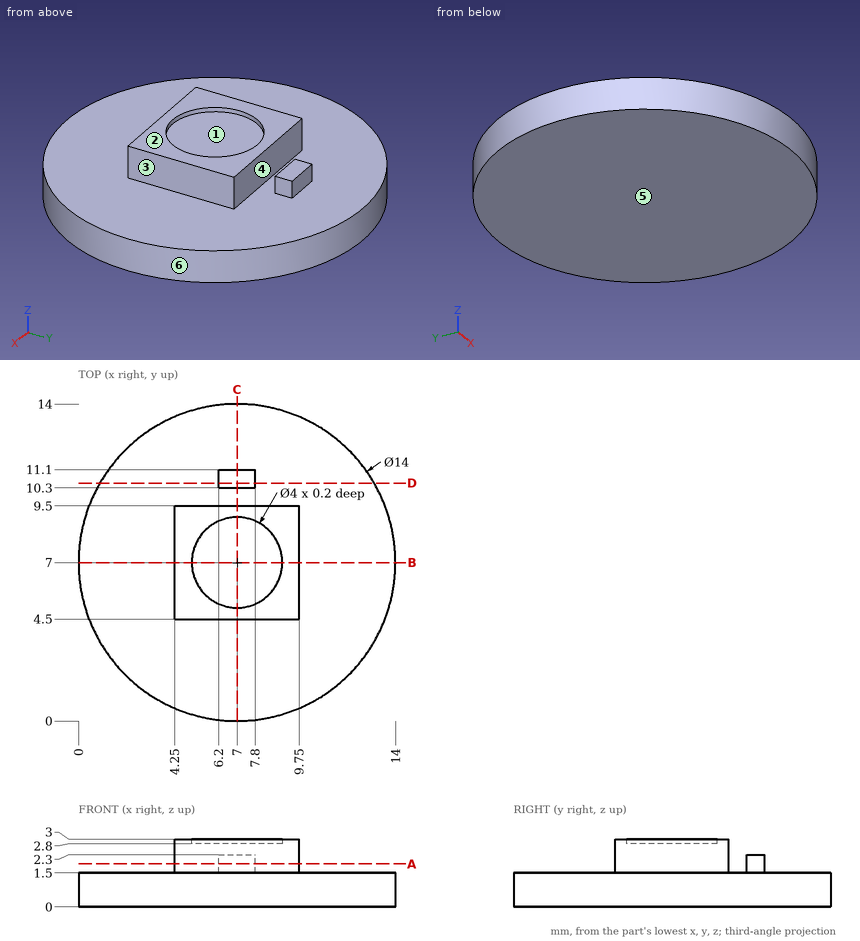
For this review, use the dimensioned drawing (mm, ordinates from the lowest corner) and the shaded views. A direction names the side the tool comes from. Round coordinates to 2 decimals unless told otherwise and drop trailing zeros. Write each loop counter-clockwise with the first axis right and the second up, starting at its lowest first coordinate (ties: lowest second). Pieces come first, ordered by that corner, then holes. Notation, with made-up numbers: M -23.75,26.5 L 10.25,26.5 A25 ccw 10.25,41.5 Z; hole C -2,-39 d11. An arc over 180 degrees is marked long. Answer as CSV lines item,"result". Start each with the question number.
Q1. The part is to be moulded in two halves that separate along Y. For the marked faces 4, 5 and 6, say which applies: +Y half, -Y half, draft (parallel to the pull), parting line (faces both ways), or undercut.
Q2. Consider section B-B, the plane y = 7. Give the boundary of the cut face in (x, z).
Q3. Consider section C-C, the plane x = 7. Give the boundary of the cut face in (y, z), then the cut area to 3 significant figures.
Q4. Clearance check with flat-ended pins moving along their axes: P1, Ø0.6, axis at y = 11, z = 2, coming from the +X side; P2, Ø0.6, axis at x = 7, z = 2, coming from the -Y side; P3, Ø1.2, axis at y = 6.5, z = 2.5, coming from the +X side. State where each tip first meets the part, or that it passes through.
Q5. Consider section D-D, the plane y = 10.5. Give the boundary of the cut face in (x, z), then the cut area to 3 significant figures.
Q6. Tool access review of the marked faces 1, 2 and 3: name each direction out of +Z, -Z, +X, -X, +Y, -Y from which nothing blocks a thin tool from reaching the whole face with its end or side.
Q7. Consider section A-A, the plane z = 1.9. Give the boundary of the cut face in (x, y).
Q8. Wall thickness on line 1 along Y through (x, z) = (7, 2.9); line 2 along Z through (x, y) = (10.75, 4.75); line 3 along X through (y, z) = (8.5, 1.6): over which ranges is each line inside the solid? List them lowest first.
Result set:
1,face 4,"undercut"
1,face 5,"draft"
1,face 6,"parting line"
2,outline,"M 0,0 L 14,0 L 14,1.5 L 9.75,1.5 L 9.75,3 L 9,3 L 9,2.8 L 5,2.8 L 5,3 L 4.25,3 L 4.25,1.5 L 0,1.5 Z"
3,outline,"M 0,0 L 14,0 L 14,1.5 L 11.1,1.5 L 11.1,2.3 L 10.3,2.3 L 10.3,1.5 L 9.5,1.5 L 9.5,3 L 9,3 L 9,2.8 L 5,2.8 L 5,3 L 4.5,3 L 4.5,1.5 L 0,1.5 Z"
3,area,"28.3 mm²"
4,P1,"stops at x = 7.8"
4,P2,"stops at y = 4.5"
4,P3,"stops at x = 9.75"
5,outline,"M 0.94,0 L 13.06,0 L 13.06,1.5 L 7.8,1.5 L 7.8,2.3 L 6.2,2.3 L 6.2,1.5 L 0.94,1.5 Z"
5,area,"19.5 mm²"
6,face 1,"+Z"
6,face 2,"+Z, +X, -X, +Y, -Y"
6,face 3,"+Z, +X, +Y, -Y"
7,outline,"M 4.25,4.5 L 9.75,4.5 L 9.75,9.5 L 4.25,9.5 Z; M 6.2,10.3 L 7.8,10.3 L 7.8,11.1 L 6.2,11.1 Z"
8,line 1,"y = 4.5 to 5, 9 to 9.5"
8,line 2,"z = 0 to 1.5"
8,line 3,"x = 4.25 to 9.75"
